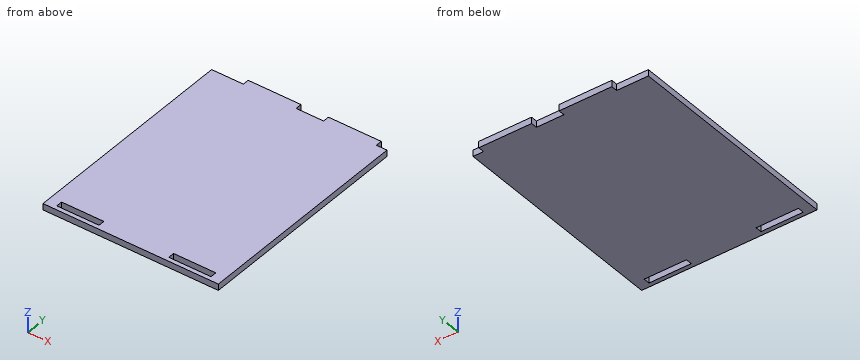
from build123d import *

# Parameters (mm, degrees)
RESSALTO_EXTRUS_O1_DEPTH = 3
ESBO_O2_W                = 20
ESBO_O2_H                = 3
CORTE_EXTRUS_O1_DEPTH    = 4


with BuildPart() as part:
    # Esboço1 → Ressalto-extrusão1 (new body)
    with BuildSketch(Plane.XY):
        Polygon((-26.514068493, 42.51552795), (-13.514068493, 42.51552795), (-13.514068493, 45.51552795), (11.485931507, 45.51552795), (11.485931507, 42.51552795), (16.485931507, 42.51552795), (16.485931507, -62.48447205), (-66.514068493, -62.48447205), (-66.514068493, 42.51552795), (-51.514068493, 42.51552795), (-51.514068493, 45.51552795), (-26.514068493, 45.51552795), align=None)
    extrude(amount=RESSALTO_EXTRUS_O1_DEPTH)

    # Esboço2 → Corte-extrusão1 (cut, through all)
    with BuildSketch(Plane(origin=(0, 0, 0), x_dir=(-1, 0, 0), z_dir=(0, 0, -1))):
        with Locations((51.514068493, -58.98447205)):
            Rectangle(ESBO_O2_W, ESBO_O2_H)
        with Locations((-1.485931507, -58.98447205)):
            Rectangle(ESBO_O2_W, ESBO_O2_H)
    extrude(amount=-CORTE_EXTRUS_O1_DEPTH, mode=Mode.SUBTRACT)


solid = part.part
Model file for the job. Use its own axes, mm. Round coordinates to 2 decimals unless told otherwise and drop trailing zeros. Loops run counter-clockwise (first coordinate to the right, second up) from the corner with the lowest first, then second, coordinate; pieces in that order, holes last. Notation, with made-up numbers: (81, 54.5) - (90, 54.5) arc R17 cw to (90, 72.5) - close; hole circle Ø9 at (-4, -29). An arc over 180 degrees is marked (long way). Write each question's results on one line, items separated by ' | '.
(1) Saw through at B-B, the plane x = -48.5. List the corners of the cut face in (y, z).
Answer below:
outline: (-62.48, 0) - (-60.48, 0) - (-60.48, 3) - (-62.48, 3) - close; (-57.48, 0) - (45.52, 0) - (45.52, 3) - (-57.48, 3) - close
(2) Wall check: L1, parallel to Y at x = 5.5, z = 1.7; L2, parallel to Y at x = -24, z = 0.75; L3, parallel to Y at x = -54, z = 2.05. Give the ranges that are in metal, low to high.
Answer below:
L1: y = -62.48 to -60.48, -57.48 to 45.52 | L2: y = -62.48 to 42.52 | L3: y = -62.48 to -60.48, -57.48 to 42.52
(3) Pin check, flat tips, straight feed: pin 1 (1.5 mm diameter, centred on y = 43.5, z = 1, fed in from +X); pin 2 (0.9 mm diameter, centred on x = -56, z = 1, fed in from +Y). Stop position of each tip, or through.
Answer below:
pin 1: stops at x = 11.49 | pin 2: stops at y = 42.52
(4) Saw through at A-A, the plane z = 1.25. List the corners of the cut face in (x, y), then the cut area to 4 significant figures.
Answer below:
outline: (-66.51, -62.48) - (16.49, -62.48) - (16.49, 42.52) - (11.49, 42.52) - (11.49, 45.52) - (-13.51, 45.52) - (-13.51, 42.52) - (-26.51, 42.52) - (-26.51, 45.52) - (-51.51, 45.52) - (-51.51, 42.52) - (-66.51, 42.52) - close; hole (-61.51, -60.48) - (-41.51, -60.48) - (-41.51, -57.48) - (-61.51, -57.48) - close; hole (-8.51, -60.48) - (11.49, -60.48) - (11.49, -57.48) - (-8.51, -57.48) - close | area: 8,745 mm^2
